Verification items for this drawing (mm, ordinates from the low corner). A direction names the side the tool comes from. Give positions to 0.01 mm unless a question says otherwise; leave off trailing zeros. Write each loop counter-clockwise with the first axis right and the second up, starting at its lowest first coordinate (ties: lowest second). Pieces come first, ordered by that corner, then holes. Notation, with made-up numbers: (-0.5, 58.5) -> (10.5, 58.5) arc R26 cw to (10.5, 90.5) -> close; hole circle Ø1 at (22, 21). An arc over 180 degrees is marked (long way). Use one line per item in the form item = value. Start each with the question number.
(1) Release check for a two-part mould opening along X. For the marked faces 1, 2 and 3 record: pulls with the +X half, pulls with the -X half, needs draft (parallel to the pull), parting line crosses it, or undercut.
(2) Section check C-C, the plane x = 62. Record the cut outline in (y, z).
(3) Scan lines: L1, parallel to X at y = 10.25, z = 15.5; L2, parallel to Y at x = 84, z = 7.5; L3, parallel to X at y = 3.25, z = 26 (1 decimal). Record each from-to range of solid material in increasing order.
(4) Set-up check for the marked faces 4 and 5: record each of +Z, -Z, +X, -X, +Y, -Y from which the full face is reachable in a straight line by a thin tool's end or side.
(5) Section check A-A, the plane y = 9.75. Record the cut outline in (x, z), plus the area to 3 significant figures.
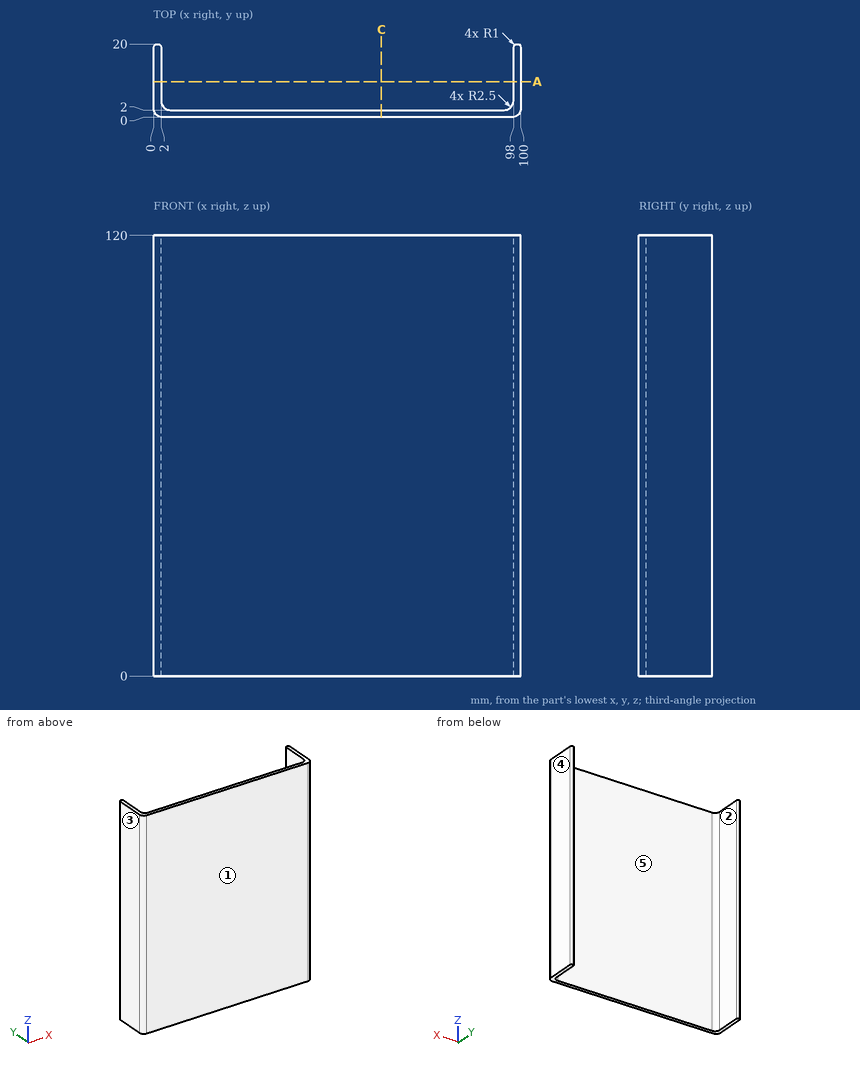
Completed:
q1.face_1 = needs draft
q1.face_2 = undercut
q1.face_3 = pulls with the -X half
q2.outline = (0, 0) -> (2, 0) -> (2, 120) -> (0, 120) -> close
q3.L1 = 0 to 2, 98 to 100
q3.L2 = 0 to 2
q3.L3 = 0 to 2.3, 97.7 to 100
q4.face_4 = +Z, -Z, +X, +Y, -Y
q4.face_5 = +Z, -Z, +Y
q5.outline = (0, 0) -> (2, 0) -> (2, 120) -> (0, 120) -> close; (98, 0) -> (100, 0) -> (100, 120) -> (98, 120) -> close
q5.area = 480 mm²
